```python
from build123d import *

# Parameters (mm, degrees)
BOSS_EXTRU_1_DEPTH      = 7.5
ENL_V_MAT_EXTRU_1_DEPTH = 25
ENL_V_MAT_EXTRU_2_DEPTH = 25


with BuildPart() as part:
    # Esquisse1 → Boss.-Extru.1 (new, symmetric)
    with BuildSketch(Plane.XY):
        Polygon((-7.5, 0), (-2.5, 0), (-2.5, 10.2), (2.5, 10.2), (2.5, 0), (7.5, 0), (7.5, 10.2), (2.5, 14.34186057), (2.5, 120), (-2.5, 120), (-2.5, 14.34186057), (-7.5, 10.2), align=None)
    extrude(amount=BOSS_EXTRU_1_DEPTH, both=True)

    # Esquisse2 → Enlèv. mat.-Extru.1 (cut)
    with BuildSketch(Plane.ZY.offset(7.5)):
        with BuildLine():
            Line((-5.164295133, 6.7), (5.164295133, 6.7))
            ThreePointArc((5.164295133, 6.7), (6.764295133, 5.1), (5.164295133, 3.5))
            Line((5.164295133, 3.5), (-5.164295133, 3.5))
            ThreePointArc((-5.164295133, 3.5), (-6.764295133, 5.1), (-5.164295133, 6.7))
        make_face()
    extrude(amount=-ENL_V_MAT_EXTRU_1_DEPTH, mode=Mode.SUBTRACT)

    # Esquisse3 → Enlèv. mat.-Extru.2 (cut)
    with BuildSketch(Plane.ZY.offset(2.5)):
        with BuildLine():
            Line((-1.6, 22.673972566), (-1.6, 111.667888004))
            ThreePointArc((-1.6, 111.667888004), (0, 113.267888004), (1.6, 111.667888004))
            Line((1.6, 111.667888004), (1.6, 22.673972566))
            ThreePointArc((1.6, 22.673972566), (0, 21.073972566), (-1.6, 22.673972566))
        make_face()
    extrude(amount=-ENL_V_MAT_EXTRU_2_DEPTH, mode=Mode.SUBTRACT)


solid = part.part
```
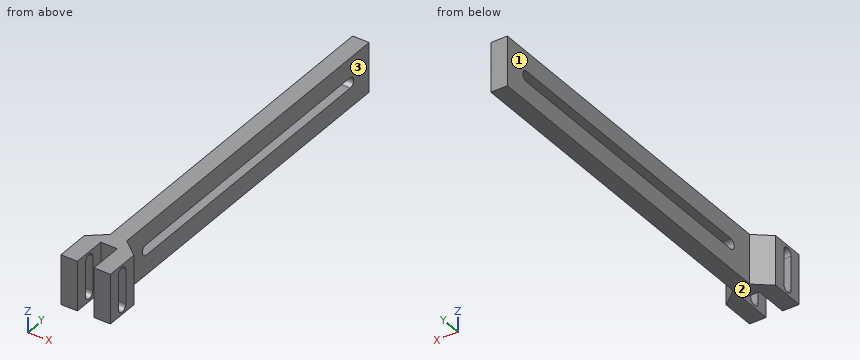
CAD build for the part. Positions are in the model's coordinates, mm. Face numbers are marked on the shaded views. A direction names the side the tool comes from. Coordinates: 2 decimals unless noted, no trailing zeros. Loops run counter-clockwise (first coordinate to the right, second up) from the corner with the lowest first, then second, coordinate; pieces in that order, holes last. Notation, with made-up numbers: (-31, 47) - (-4, 47) arc R27 cw to (-4, 81) - close; hole circle Ø7 at (-9.75, -39). An arc over 180 degrees is marked (long way). Return JSON: item names as keys, results as strings.
1. 3-axis set-ups, long thin cutter, end or side, ignore diameter. For the marked faces 1, 2 and 3: which of +Z, -Z, +X, -X, +Y, -Y reach the whole face in a straight line?
Result:
{"face 1": "+Z, -Z, -X, +Y", "face 2": "-Z, +X, -X, +Y, -Y", "face 3": "+Z, -Z, +X, +Y"}
2. Band-saw the part on B-B (z = 0). Give the cut face in (x, y).
Result:
{"outline": "(-7.5, 0) - (-2.5, 0) - (-2.5, 3.5) - (-7.5, 3.5) - close; (-7.5, 6.7) - (-2.5, 6.7) - (-2.5, 10.2) - (2.5, 10.2) - (2.5, 6.7) - (7.5, 6.7) - (7.5, 10.2) - (2.5, 14.34) - (2.5, 21.07) - (-2.5, 21.07) - (-2.5, 14.34) - (-7.5, 10.2) - close; (-2.5, 113.27) - (2.5, 113.27) - (2.5, 120) - (-2.5, 120) - close; (2.5, 0) - (7.5, 0) - (7.5, 3.5) - (2.5, 3.5) - close"}
3. Band-saw the part on D-D (y = 99.5). Give the cut face in (x, z), and give its area (3 significant figures).
Result:
{"outline": "(-2.5, -7.5) - (2.5, -7.5) - (2.5, -1.6) - (-2.5, -1.6) - close; (-2.5, 1.6) - (2.5, 1.6) - (2.5, 7.5) - (-2.5, 7.5) - close", "area": "59.0 mm2"}
4. Band-saw the part on C-C (x = 1.5). Give the cut face in (y, z), and give its area (3 significant figures).
Result:
{"outline": "(10.2, -7.5) - (120, -7.5) - (120, 7.5) - (10.2, 7.5) - close; hole (22.67, -1.6) - (111.67, -1.6) arc R1.6 ccw to (111.67, 1.6) - (22.67, 1.6) arc R1.6 ccw to start", "area": "1,350 mm2"}
5. Band-saw the part on A-A (y = 5.1). Give the cut face in (x, z).
Result:
{"outline": "(-7.5, -7.5) - (-2.5, -7.5) - (-2.5, -6.76) - (-7.5, -6.76) - close; (-7.5, 6.76) - (-2.5, 6.76) - (-2.5, 7.5) - (-7.5, 7.5) - close; (2.5, -7.5) - (7.5, -7.5) - (7.5, -6.76) - (2.5, -6.76) - close; (2.5, 6.76) - (7.5, 6.76) - (7.5, 7.5) - (2.5, 7.5) - close"}
6. Drop flat-ended pins along their axis: pin 1 (2 mm diameter, centred on x = -5, z = 4.5, fed in from +Y); pin 2 (1.5 mm diameter, centred on x = -1, z = 3, fed in from -Y); pin 3 (5 mm diameter, centred on y = 15, z = -5.5, fed in from -X). Give the stop position or say it passes through.
Result:
{"pin 1": "stops at y = 13.1", "pin 2": "stops at y = 10.2", "pin 3": "stops at x = -4.72"}
7. Probe L1, parallel to Z at x = 0.75, y = 106.5; L2, parallel to X at y = 96, z = -3.25; L3, parallel to Y at x = 3, z = 2.5. List the from-to ranges inside material, lowest first. Write a range as from..to.
Result:
{"L1": "z = -7.5..-1.6, 1.6..7.5", "L2": "x = -2.5..2.5", "L3": "y = 0..3.5, 6.7..13.93"}
